Check sheet for the modelled part. Datum: model origin and axes. Units: mm. A direction names the side the tool comes from. Round coordinates to 2 decimals unless told otherwise and drop trailing zeros. Write each loop counter-clockwise with the first axis right and the second up, starting at its lowest first coordinate (ties: lowest second). Pieces come first, ordered by that corner, then holes.
Item 1: Material ranges on line 1 along X through (y, z) = (3.5, 7); line 2 along Y through (x, z) = (-0.5, 1.5); line 3 along Z through (x, y) = (-3, -17.5), recorded low to high.
Item 2: Set-up check for faces 1 (the cylindrical face through (0.045, 6.476, 8.777)), 2 (the cylindrical face through (2.285, 3.584, 5.324)): record each of +Z, -Z, +X, -X, +Y, -Y from which the full face is reachable in a straight line by a thin tool's end or side.
Item 3: Section check B-B, the plane z = 9. State how many separate pieces and enclosed holes the cut face has, plus the area to 3 significant figures.
Item 4: Release check for a two-part mould opening along Y. For faces 3 (the cylindrical face through (4.336, 19.524, 4.93)), 4 (the flat face through (4.3, 2.4, 11)), 5 (the conical face through (4.2, -4.4, 6.1)) record: pulls with the +Y half, pulls with the -Y half, needs draft (parallel to the pull), parting line crosses it, or undercut.
Item 5: Depth check by flat-ended pin: pin 1 (4 mm diameter, centred on y = -11, z = 2, fed in from -X); pin 2 (1.5 mm diameter, centred on x = -9, y = -12, fed in from +Z); pin 3 (4 mm diameter, centred on y = -7.5, z = 2, fed in from -X); pin 4 (3 mm diameter, centred on x = -2.5, y = -1, fed in from -Z). Enter the tip coordinate at first touch or a pass-through.
Item 6: Section check A-A, the plane z = 4.25. Record the cut outline in (x, y).
from build123d import *

# Parameters (mm, degrees)
SKETCH1_R                    = 20
BOSS_EXTRUDE1_DEPTH          = 10.5
SKETCH2_R                    = 10.5
SKETCH2_R_2                  = 4.25
BOSS_EXTRUDE3_DEPTH          = 0.5
BOSS_EXTRUDE3_DRAFT          = 45
SKETCH3_R                    = 4.25
CUT_EXTRUDE1_DEPTH           = 10.5
M2_5X0_45_TAPPED_HOLE1_D     = 2.05
M2_5X0_45_TAPPED_HOLE1_DEPTH = 4.384117865
M2_5X0_45_TAPPED_HOLE1_TIP   = 0.615882135
FILLET1_R                    = 0.5


with BuildPart() as part:
    # Sketch1 → Boss-Extrude1 (new body)
    with BuildSketch(Plane(origin=(0, 0, 0), x_dir=(0, 1, 0), z_dir=(0, 0, 1))):
        with Locations(Location((0, 0, 0), (0, 0, 90))):
            Circle(SKETCH1_R)
    extrude(amount=BOSS_EXTRUDE1_DEPTH)


with BuildPart() as boss_extrude3_tool:
    # Sketch2 → Boss-Extrude3 (with draft: the straight prism first)
    with BuildSketch(Plane.XY.offset(10.5)):
        Circle(SKETCH2_R)
        Circle(SKETCH2_R_2, mode=Mode.SUBTRACT)
    extrude(amount=BOSS_EXTRUDE3_DEPTH)
    # Boss-Extrude3: the draft: its side faces are tilted about the plane it starts from
    boss_extrude3_sides = [boss_extrude3_tool.faces().sort_by_distance(p)[0] for p in [
        (-10.5, 0, 10.75),
        (-4.25, 0, 10.75),
    ]]
    draft(boss_extrude3_sides, Plane.XY.offset(10.5), BOSS_EXTRUDE3_DRAFT)


with BuildPart() as part_1:
    add(part.part)

    # Boss-Extrude3: add boss_extrude3_tool
    add(boss_extrude3_tool.part)

    # Sketch3 → Cut-Extrude1 (cut)
    with BuildSketch(Plane.XY.offset(10.5)):
        Circle(SKETCH3_R)
    extrude(amount=-CUT_EXTRUDE1_DEPTH, mode=Mode.SUBTRACT)

    # M2.5x0.45 Tapped Hole1
    with Locations(Plane(origin=(0, 0, 11), x_dir=(0, -1, 0), z_dir=(0, 0, 1))):
        with Locations((4.242640687, -4.242640687), (-7.5, 0), (0, -7.5), (7.5, 0), (0, 7.5), (4.242640687, 4.242640687), (-4.242640687, 4.242640687), (-4.242640687, -4.242640687)):
            Hole(M2_5X0_45_TAPPED_HOLE1_D / 2, depth=M2_5X0_45_TAPPED_HOLE1_DEPTH)
            with Locations((0, 0, -(M2_5X0_45_TAPPED_HOLE1_DEPTH + M2_5X0_45_TAPPED_HOLE1_TIP / 2))):  # 118° drill point
                Cone(0, M2_5X0_45_TAPPED_HOLE1_D / 2, M2_5X0_45_TAPPED_HOLE1_TIP, mode=Mode.SUBTRACT)

    # Fillet1
    fillet1_edges = [part_1.edges().sort_by_distance(p)[0] for p in [
        (20, 0, 10.5),
    ]]
    fillet(fillet1_edges, radius=FILLET1_R)


solid = part_1.part
Values found:
1. line 1: x = -19.69 to -4.95, -3.54 to -2.41, 2.41 to 3.54, 4.95 to 19.69
1. line 2: y = -19.99 to -4.22, 4.22 to 19.99
1. line 3: z = 0 to 10.5
2. face 1: +Z
2. face 2: +Z, -Z
3. separate pieces: 1
3. enclosed holes: 9
3. area: 1,170 mm2
4. face 3: parting line crosses it
4. face 4: needs draft
4. face 5: undercut
5. pin 1: stops at x = -17.86
5. pin 2: stops at z = 10.5
5. pin 3: stops at x = -19.23
5. pin 4: passes through
6. outline: circle Ø40 at (0, 0); hole circle Ø8.5 at (0, 0)
